from build123d import *

# Parameters (mm, degrees)
ESQUISSE1_R             = 17.5
BOSS_EXTRU_1_DEPTH      = 26
CONG_1_R                = 3
ESQUISSE2_R             = 2
BOSS_EXTRU_2_DEPTH      = 20
ESQUISSE3_R             = 2.5
BOSS_EXTRU_3_DEPTH      = 5
CONG_5_R                = 1
ESQUISSE6_R             = 4.037593864
ENL_V_MAT_EXTRU_1_DEPTH = 7
ESQUISSE7_R             = 1.25
BOSS_EXTRU_4_DEPTH      = 3
ESQUISSE9_R             = 1.25
BOSS_EXTRU_5_DEPTH      = 3
ESQUISSE10_R            = 1.25
BOSS_EXTRU_6_DEPTH      = 3
ESQUISSE11_R            = 1.25
BOSS_EXTRU_7_DEPTH      = 3
ESQUISSE12_R            = 7.076094554
ENL_V_MAT_EXTRU_3_DEPTH = 32


with BuildPart() as part:
    # Esquisse1 → Boss.-Extru.1 (new body)
    with BuildSketch(Plane.XY):
        with Locations(Location((0, 0, 0), (0, 0, 180))):
            Circle(ESQUISSE1_R)
    extrude(amount=BOSS_EXTRU_1_DEPTH)

    # Congé1
    cong_1_edges = [part.edges().sort_by_distance(p)[0] for p in [
        (17.5, 0, 0),
        (17.5, 0, 26),
    ]]
    fillet(cong_1_edges, radius=CONG_1_R)

    # Esquisse2 → Boss.-Extru.2 (add)
    with BuildSketch(Plane.XY.offset(26)):
        Circle(ESQUISSE2_R)
    extrude(amount=BOSS_EXTRU_2_DEPTH)

    # Esquisse3 → Boss.-Extru.3 (add)
    with BuildSketch(Plane(origin=(0, 0, 0), x_dir=(-1, 0, 0), z_dir=(0, 0, -1))):
        with Locations(Location((0, 0, 0), (0, 0, 180))):
            Circle(ESQUISSE3_R)
    extrude(amount=BOSS_EXTRU_3_DEPTH)

    # Congé5
    cong_5_edges = [part.edges().sort_by_distance(p)[0] for p in [
        (-2.5, 0, -5),
    ]]
    fillet(cong_5_edges, radius=CONG_5_R)

    # Lissage1: read off the stored shape, not the designer's step
    # Lissage1: loft between two sections, ruled curve by curve
    lissage1_from = [
        Edge.make_bspline([(-1.703307527, 1.048209649, 26), (-3.799726825, -2.358405406, 26), (-0.39311177, -4.454824703, 26), (1.703307527, -1.048209649, 26), (3.799726825, 2.358405406, 26), (0.39311177, 4.454824703, 26), (-1.703307527, 1.048209649, 26)], [0, 0, 0, 0, 0.5, 0.5, 0.5, 1, 1, 1, 1], 3, [1, 0.333333333, 0.333333333, 1, 0.333333333, 0.333333333, 1]),
    ]
    lissage1_to = [
        Edge.make_bspline([(5.264402681, 2.231137224, 33), (0.802128233, 12.759942587, 33), (-9.72667713, 8.297668139, 33), (-5.264402681, -2.231137224, 33), (-0.802128233, -12.759942587, 33), (9.72667713, -8.297668139, 33), (5.264402681, 2.231137224, 33)], [0, 0, 0, 0, 0.5, 0.5, 0.5, 1, 1, 1, 1], 3, [1, 0.333333333, 0.333333333, 1, 0.333333333, 0.333333333, 1]),
    ]
    lissage1 = Solid(Shell([*[Face.make_surface_from_curves(lissage1_from[k], lissage1_to[k]) for k in range(1)], Face(Wire(lissage1_from)), Face(Wire(lissage1_to))]))
    add(lissage1)

    # Esquisse6 → Enlèv. mat.-Extru.1 (cut)
    with BuildSketch(Plane.XY.offset(46)):
        Circle(ESQUISSE6_R)
    extrude(amount=-ENL_V_MAT_EXTRU_1_DEPTH, mode=Mode.SUBTRACT)

    # Esquisse7 → Boss.-Extru.4 (add)
    with BuildSketch(Plane(origin=(0, 0, 0), x_dir=(-1, 0, 0), z_dir=(0, 0, -1))):
        with BuildLine():
            Line((4, 0), (4, -25))
            ThreePointArc((4, -25), (0, -29), (-4, -25))
            Line((-4, -25), (-4, 0))
            ThreePointArc((-4, 0), (0, 4), (4, 0))
        make_face()
        with Locations((0, -25)):
            Circle(ESQUISSE7_R, mode=Mode.SUBTRACT)
    extrude(amount=BOSS_EXTRU_4_DEPTH)

    # Esquisse9 → Boss.-Extru.5 (add)
    with BuildSketch(Plane(origin=(0, 0, 0), x_dir=(-1, 0, 0), z_dir=(0, 0, -1))):
        with BuildLine():
            Line((-4, 0), (-4, 25))
            ThreePointArc((-4, 25), (0, 29), (4, 25))
            Line((4, 25), (4, 0))
            ThreePointArc((4, 0), (0, -4), (-4, 0))
        make_face()
        with Locations((0, 25)):
            Circle(ESQUISSE9_R, mode=Mode.SUBTRACT)
    extrude(amount=BOSS_EXTRU_5_DEPTH)

    # Esquisse10 → Boss.-Extru.6 (add)
    with BuildSketch(Plane(origin=(0, 0, 0), x_dir=(-1, 0, 0), z_dir=(0, 0, -1))):
        with BuildLine():
            Line((0, -4), (-25, -4))
            ThreePointArc((-25, -4), (-29, 0), (-25, 4))
            Line((-25, 4), (0, 4))
            ThreePointArc((0, 4), (4, 0), (0, -4))
        make_face()
        with Locations((-25, 0)):
            Circle(ESQUISSE10_R, mode=Mode.SUBTRACT)
    extrude(amount=BOSS_EXTRU_6_DEPTH)

    # Esquisse11 → Boss.-Extru.7 (add)
    with BuildSketch(Plane(origin=(0, 0, 0), x_dir=(-1, 0, 0), z_dir=(0, 0, -1))):
        with BuildLine():
            Line((0, 4), (25, 4))
            ThreePointArc((25, 4), (29, 0), (25, -4))
            Line((25, -4), (0, -4))
            ThreePointArc((0, -4), (-4, 0), (0, 4))
        make_face()
        with Locations((25, 0)):
            Circle(ESQUISSE11_R, mode=Mode.SUBTRACT)
    extrude(amount=BOSS_EXTRU_7_DEPTH)

    # Esquisse12 → Enlèv. mat.-Extru.3 (cut)
    with BuildSketch(Plane(origin=(0, 0, -3), x_dir=(-1, 0, 0), z_dir=(0, 0, -1))):
        Circle(ESQUISSE12_R)
    extrude(amount=ENL_V_MAT_EXTRU_3_DEPTH, mode=Mode.SUBTRACT)


solid = part.part
Model file for the job. Use its own axes, mm. A direction names the side the tool comes from. Give positions to 0.01 mm unless a question says otherwise; leave off trailing zeros. Order: outer loops, then holes, each group sorted by start corner. A loop starts at its lowest first (then second) coordinate and runs counter-clockwise, first axis right, second up. Notation, with made-up numbers: (70, -38.75) - (112, -38.75) arc R17 ccw to (112, -7.75) - close; hole circle Ø3 at (47, 30.25). An arc over 180 degrees is marked (long way). Write item = value, one per line. Start each with the question number.
1. Cut at A-A, the plane x = 0. State how many separate pieces and enclosed holes the cut face has, and give its area (3 significant figures).
2. Two-plate mould, pull along Y, no slides. Class faces 1 (the cylindrical face through (0, -29, -1)), 2 (the cylindrical face through (-26.155, -0.479, -1.479)), 3 (the cylindrical face through (23.845, -0.479, -1.479)), 4 (the flat face through (-4, -14, -1)): pulls with the +Y half, pulls with the -Y half, needs draft (parallel to the pull), parting line crosses it, or undercut.
3. Cut at B-B, the plane z = 14. List the corners of the cut face in (x, y), and give its area (3 significant figures).
4. Probe line 1 along Y through (x, z) = (0, -1.9); line 2 along Y through (x, z) = (-25, -1.4); line 3 along Z through (x, y) = (18.5, 2). List the from-to ranges inside material, lowest first.
5. Cut at D-D, the plane y = 19.5. List the corners of the cut face in (x, z), and give its area (3 significant figures).
6. Which spindle directions (+Z, -Z, +X, -X, +Y, -Y) get a long thin tool onto all of the face, cutting with end or side? Do faces 5 (the flat face through (15, 4, -1)), 6 (the flat face through (0, 0, -3)), 7 (the flat face through (-4, 15, -1)), 8 (the cylindrical face through (0, 29, -1)), 9 (the flat face through (-2.2, -0.1, 33)). Say none if no direction does.
7. Drop flat-ended pins along their axis: P1, Ø1.5, axis at y = -15, z = -2, coming from the -X side; P2, Ø8, axis at x = 7.5, y = -10, coming from the -Z side; P3, Ø8, axis at x = 10, y = 10, coming from the -Z side; P4, Ø1, axis at y = 16.5, z = 10, coming from the +X side. Give the stop position or say it passes through.
Taken from the geometry:
q1.separate_pieces = 3
q1.enclosed_holes = 0
q1.area = 1,130 mm²
q2.face_1 = pulls with the -Y half
q2.face_2 = undercut
q2.face_3 = undercut
q2.face_4 = needs draft
q3.outline = circle Ø35 at (0, 0)
q3.area = 962 mm²
q4.line_1 = -29 to -26.25, -23.75 to 23.75, 26.25 to 29
q4.line_2 = -4 to -1.25, 1.25 to 4
q4.line_3 = -3 to 0
q5.outline = (-4, -3) - (4, -3) - (4, 0) - (-4, 0) - close
q5.area = 24.0 mm²
q6.face_5 = -Z, +X, +Y
q6.face_6 = -Z, +X, -X, +Y, -Y
q6.face_7 = -Z, -X, +Y
q6.face_8 = +Z, -Z, +Y
q6.face_9 = +Z
q7.P1 = -4
q7.P2 = -3
q7.P3 = 0
q7.P4 = 7.09
